Answer from the drawing. Dimensions are ordinates in mm from the lowest x, y and z of the part. A direction names the side the tool comes from. Round coordinates to 2 decimals unless told otherwise and drop trailing zeros. Write each loop counter-clockwise with the first axis right and the second up, starting at its lowest first coordinate (ties: lowest second). Pieces come first, ordered by that corner, then holes.
1. Flat-ended cylindrical pins translate along their axes: pin 1 Ø2 at (x, y) = (5.5, 5) entering from +Z (3 decimals); pin 2 Ø2 at (y, z) = (9.5, 2) entering from +X; pin 3 Ø8 at (x, y) = (8.5, 2.5) entering from -Z (3 decimals); pin 4 Ø2 at (x, y) = (15, 10) entering from +Z. Find the tip coordinate at first contact, or state that the pin passes through.
2. Determine the mould class of the marked faces 1, 2, 3 and 4 for opening direction X: pulls with the +X half, pulls with the -X half, needs draft (parallel to the pull), parting line crosses it, or undercut.
3. Straight lines are drawn through the part: probe 1 along Y at (x, z) = (11.1, 12.5); probe 2 along Y at (x, z) = (17.5, 15); probe 3 along Z at (x, y) = (4.75, 19) (3 decimals). For each, find the intervals that lie inside material, in ascending order.
4. Find section C-C (z = 16.25). Write down the section's boundary in (x, y).
5. Find section D-D (x = 6.25). Write down the section's boundary in (y, z) (1 decimal).
6. A tool of negligible diameter and unlimited length cuts with its end or side. For the marked faces 5, 6 and 7, from which of +Z, -Z, +X, -X, +Y, -Y can it reach the whole face along a straight path? Write none if from no direction.
7. Find section A-A (y = 11.1). Write down the section's boundary in (x, z) (3 decimals).
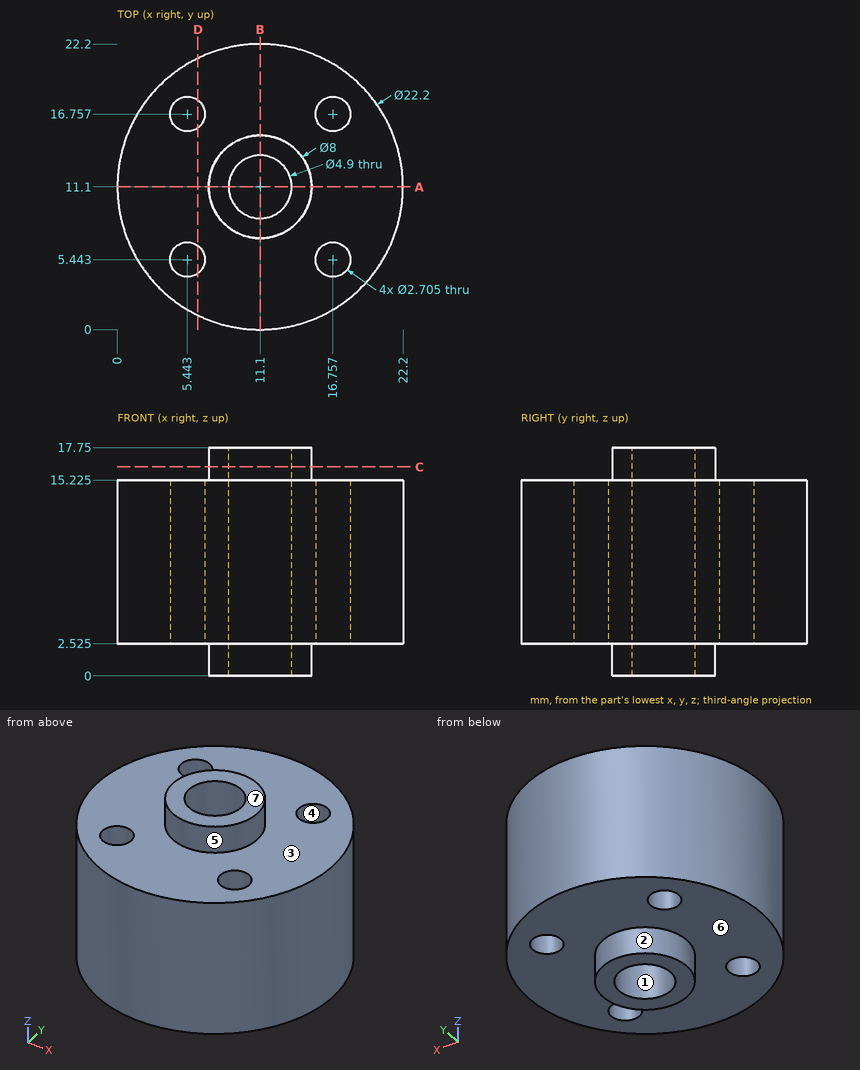
Worked answers:
1. pin 1: stops at z = 15.225
1. pin 2: stops at x = 22.17
1. pin 3: stops at z = 2.525
1. pin 4: stops at z = 17.75
2. face 1: undercut
2. face 2: parting line crosses it
2. face 3: needs draft
2. face 4: undercut
3. probe 1: y = 0 to 8.65, 13.55 to 22.2
3. probe 2: y = 2.03 to 4.31, 6.57 to 15.63, 17.89 to 20.17
3. probe 3: z = 2.525 to 15.225
4. outline: circle Ø8 at (11.1, 11.1); hole circle Ø4.9 at (11.1, 11.1)
5. outline: (1.1, 2.5) - (4.4, 2.5) - (4.4, 15.2) - (1.1, 15.2) - close; (6.5, 2.5) - (15.7, 2.5) - (15.7, 15.2) - (6.5, 15.2) - close; (17.8, 2.5) - (21.1, 2.5) - (21.1, 15.2) - (17.8, 15.2) - close
6. face 5: +Z
6. face 6: -Z
6. face 7: +Z, +X, -X, +Y, -Y
7. outline: (0, 2.525) - (7.1, 2.525) - (7.1, 0) - (8.65, 0) - (8.65, 17.75) - (7.1, 17.75) - (7.1, 15.225) - (0, 15.225) - close; (13.55, 0) - (15.1, 0) - (15.1, 2.525) - (22.2, 2.525) - (22.2, 15.225) - (15.1, 15.225) - (15.1, 17.75) - (13.55, 17.75) - close
